Design review of the part built by this model. Coordinates are the model's own, in mm. A direction names the side the tool comes from. Give positions to 0.01 mm unless a question says otherwise; leave off trailing zeros. Order: outer loops, then holes, each group sorted by start corner. A loop starts at its lowest first (then second) coordinate and runs counter-clockwise, first axis right, second up. Notation, with made-up numbers: (60, -11.75) -> (64, -11.75) arc R21 ccw to (64, 6.25) -> close; hole circle Ø4 at (11.5, 52). An arc over 180 degrees is marked (long way). Return JSON: item names as keys, results as strings.
Autodesk Inventor part; units mm, degrees
ref_plane "YZ Plane" through (0, 0, 0) normal (1, 0, 0) x (0, 1, 0)
ref_plane "XZ Plane" through (0, 0, 0) normal (0, 1, 0) x (-1, 0, 0)
ref_plane "XY Plane" through (0, 0, 0) normal (0, 0, 1) x (1, 0, 0)
sketch "Sketch1" plane through (0, 0, 0) normal (0, 1, 0) x (-1, 0, 0)
  line L0 (0, 0) -> (-92, 0)
  line L1 (-92, 0) -> (-92, -88)
  line L2 (-92, -88) -> (0, -88)
  line L3 (0, -88) -> (0, 0)
  line L4 (0, -88) -> (-5, -88)
  line L5 (-5, -88) -> (-5, -85)
  line L6 (-5, -85) -> (0, -85)
  line L7 (0, -85) -> (0, -88)
  line L8 (0, 0) -> (-5, 0)
  line L9 (-5, 0) -> (-5, -3)
  line L10 (-5, -3) -> (0, -3)
  line L11 (0, -3) -> (0, 0)
  line L12 (-92, 0) -> (-87, 0)
  line L13 (-87, 0) -> (-87, -3)
  line L14 (-87, -3) -> (-92, -3)
  line L15 (-92, -3) -> (-92, 0)
  line L16 (-92, -88) -> (-87, -88)
  line L17 (-87, -88) -> (-87, -85)
  line L18 (-87, -85) -> (-92, -85)
  line L19 (-92, -85) -> (-92, -88)
  circle A0 centre (-9, -84) radius 1.6 construction
  circle A1 centre (-83, -84) radius 1.6 construction
  circle A2 centre (-9, -4) radius 1.6 construction
  circle A3 centre (-83, -4) radius 1.6 construction
  circle A4 centre (-46, -85) radius 1.6 construction
  circle A5 centre (-3, -44) radius 1.6 construction
  circle A6 centre (-89, -44) radius 1.6 construction
  circle A7 centre (-46, -3) radius 1.6 construction
  circle A8 centre (-9, -84) radius 3
  circle A9 centre (-46, -85) radius 3
  circle A10 centre (-83, -84) radius 3
  circle A11 centre (-3, -44) radius 3
  circle A12 centre (-9, -4) radius 3
  circle A13 centre (-83, -4) radius 3
  circle A14 centre (-89, -44) radius 3
  circle A15 centre (-46, -3) radius 3
  line L20 (-11.8284, -3) -> (-43, -3)
  line L21 (-49, -3) -> (-80.1716, -3)
  line L22 (-83, -7) -> (-89, -7)
  line L23 (-89, -7) -> (-89, -41)
  line L24 (-83, -81) -> (-89, -81)
  line L25 (-89, -81) -> (-89, -47)
  line L26 (-80.1716, -85) -> (-49, -85)
  line L27 (-43, -85) -> (-11.8284, -85)
  line L28 (-9, -81) -> (-3, -81)
  line L29 (-9, -7) -> (-3, -7)
  line L30 (-3, -7) -> (-3, -41)
  line L31 (-3, -47) -> (-3, -81)
  point P0 (-92, -44)
  point P1 (-46, 0)
  dimension "d0" = 82
  dimension "d1" = 88
  dimension "d2" = 92
  dimension "d3" = 5
  dimension "d4" = 3.2
  dimension "d5" = 74
  dimension "d6" = 80
  dimension "d7" = 9
  dimension "d8" = 4
  dimension "d9" = 3.2
  dimension "d10" = 46
  dimension "d11" = 44
  dimension "d12" = 3
  dimension "d13" = 3
  dimension "d14" = 3
  dimension "d15" = 3
  dimension "d16" = 6
  dimension "d17" = 3
  dimension "d18" = 3
  dimension "d19" = 3
  dimension "d20" = 3
extrude "Extrusion1" add sketch "Sketch1" along normal blind 5 contours L9 L10 L3 A11 L30 L29 A12 L20 A15 L0 | A15 L21 A13 L22 L23 A14 L1 L14 L13 L0 | A15 | A11 | L3 L6 L5 L2 A9 L27 A8 L28 L31 A11 | A12 | A13 | A8 | A14 L25 L24 A10 L26 A9 L2 L17 L18 L1 | A14 | A9 | A10
fillet "Fillet1" radius 3 16 edges at (3, 2.5, -7) (11.8284, 2.5, -3) (43, 2.5, -3) (49, 2.5, -3) (80.1716, 2.5, -3) (89, 2.5, -7) (89, 2.5, -41) (89, 2.5, -47) (3, 2.5, -41) (3, 2.5, -47) (3, 2.5, -81) (11.8284, 2.5, -85) (43, 2.5, -85) (49, 2.5, -85) (89, 2.5, -81) (80.1716, 2.5, -85)
sketch "Sketch2" plane through (0, 5, 0) normal (0, 1, 0) x (1, 0, 0)
  arc A0 (87.5, 46.5981) -> (87.5, 41.4019) centre (89, 44) ccw
  arc A1 (43.4019, 83.5) -> (48.5981, 83.5) centre (46, 85) ccw
  arc A2 (4.5, 41.4019) -> (4.5, 46.5981) centre (3, 44) ccw
  arc A3 (48.5981, 4.5) -> (43.4019, 4.5) centre (46, 3) ccw
  point P0 (0, 0)
  point P1 (92, 44)
  point P2 (46, 0)
hole "Hole1" at (46, 5, -85) at (3, 5, -44) at (89, 5, -44) at (46, 5, -3) direction (0, -1, 0) diameter 2.459 end through all
sketch "Sketch3" plane through (0, 5, 0) normal (0, 1, 0) x (1, 0, 0)
  arc A0 (9, 81) -> (11.8284, 83) centre (9, 84) ccw
  arc A1 (11.8284, 5) -> (9, 7) centre (9, 4) ccw
  arc A2 (80.1716, 83) -> (83, 81) centre (83, 84) ccw
  arc A3 (83, 7) -> (80.1716, 5) centre (83, 4) ccw
  point P0 (0, 0)
  point P1 (84, 6)
hole "Hole2" at (9, 5, -84) at (9, 5, -4) at (83, 5, -4) at (83, 5, -84) direction (0, -1, 0) diameter 3.2 end through all
equation "\"d7\" = -0.5 * d5 + 0.5 * d2"
equation "\"d8\" = -0.5 * d6 + 0.5 * d1"
equation "\"d10\" = 0.5 * d2"
equation "\"d11\" = 0.5 * d1"
equation "\"d13\" = d12"
equation "\"d15\" = d14"
equation "\"d17\" = d19"
equation "\"d18\" = d20"
properties part number "ElectronicsBayUpperMount"
Item 1: Add section A-A (x = 56). Give the boundary of the cut face in (y, z).
Result set:
{"outline": "(0, -88) -> (5, -88) -> (5, -85) -> (0, -85) -> close; (0, -3) -> (5, -3) -> (5, 0) -> (0, 0) -> close"}
Item 2: Machinability: for faces 4 (the face through (89, 2, -85)), 5 (the face through (88.1, 2.54, -7.86)), 6 (the face through (46, 5, -5)), 7 (the face through (45, 2, 0)), 8 (the face through (3, 2, -85)), which of the approach directions +Z, -Z, +X, -X, +Y, -Y give a long, thin tool a straight path to every point of the face, cutting with its end or side? Answer none if there is none.
Result set:
{"face 4": "-Z, +X, +Y, -Y", "face 5": "+Y, -Y", "face 6": "+Z, -Z, +X, -X, +Y", "face 7": "+Z, +X, -X, +Y, -Y", "face 8": "-Z, -X, +Y, -Y"}
Item 3: Add section B-B (z = -33). Give the boundary of the cut face in (x, y), plus the area to 3 significant figures.
Result set:
{"outline": "(0, 0) -> (3, 0) -> (3, 5) -> (0, 5) -> close; (89, 0) -> (92, 0) -> (92, 5) -> (89, 5) -> close", "area": "30.0 mm^2"}
Item 4: Add section C-C (y = 3.6). Give the number of separate pieces and of enclosed holes in the cut face, plus the area to 3 significant figures.
Result set:
{"separate pieces": "1", "enclosed holes": "9", "area": "1,140 mm^2"}
Item 5: Wall thickness on L1, parallel to Z at x = 9, y = 3.8; L2, parallel to X at y = 0.3, z = -15.5; L3, parallel to Z at x = 46, y = 2.1: over which ranges is each line inside the solid? List them lowest first. Write a range as [from, to].
Result set:
{"L1": "z = [-88, -85.6], [-82.4, -81], [-7, -5.6], [-2.4, 0]", "L2": "x = [0, 3], [89, 92]", "L3": "z = [-88, -86.23], [-83.77, -82], [-6, -4.23], [-1.77, 0]"}
Item 6: Mouldability with a two-part tool opening along X and no side actions: class faces 1 (the face through (5, 2, -1)), 2 (the face through (46, 0, -5)), 3 (the face through (8.93, 2.46, -85.6)) as released by +X, released by -X, zero draft, split by the parting line, or undercut.
Result set:
{"face 1": "released by -X", "face 2": "zero draft", "face 3": "undercut"}
Item 7: For pin 1 (1.5 mm diameter, centred on x = 89, y = 3, fed in from -Z); pin 2 (3 mm diameter, centred on x = 9, z = -84, fed in from +Y); pin 3 (1.5 mm diameter, centred on y = 2.5, z = -2, fed in from -X), all flat-tipped, find the tip position at first contact; note any pin that passes through.
Result set:
{"pin 1": "stops at z = -85", "pin 2": "passes through", "pin 3": "stops at x = 5"}
